The drawing under review shows one solid part. Ordinate dimensions are in mm from its lowest x, y, z. A direction names the side the tool comes from. Coordinates: 2 decimals unless noted, no trailing zeros. Write each loop counter-clockwise with the first axis right and the second up, starting at its lowest first coordinate (ties: lowest second). Pieces come first, ordered by that corner, then holes.
1) For line 1 (Y direction, x = 3.8, z = 5.4); line 2 (X direction, y = 5.25, z = 2.9); line 3 (Y direction, x = 1.3, z = 2.45), list the stretches that pass through material, from the lowest coordinate up.
2) Machinability: for the marked faces 1 and 2, which of the approach directions +Z, -Z, +X, -X, +Y, -Y give a long, thin tool a straight path to every point of the face, cutting with its end or side? Answer none if there is none.
3) Add section A-A, the plane y = 3.5. State the section outline as (x, z) points.
4) For P1, Ø1, axis at y = 7, z = 0.5, coming from the -X side; P2, Ø3, axis at x = 2, z = 4.5, coming from the -Y side; P3, Ø2, axis at x = 3, y = 7.5, coming from the +Z side, all flat-tipped, find the tip position at first contact; note any pin that passes through.
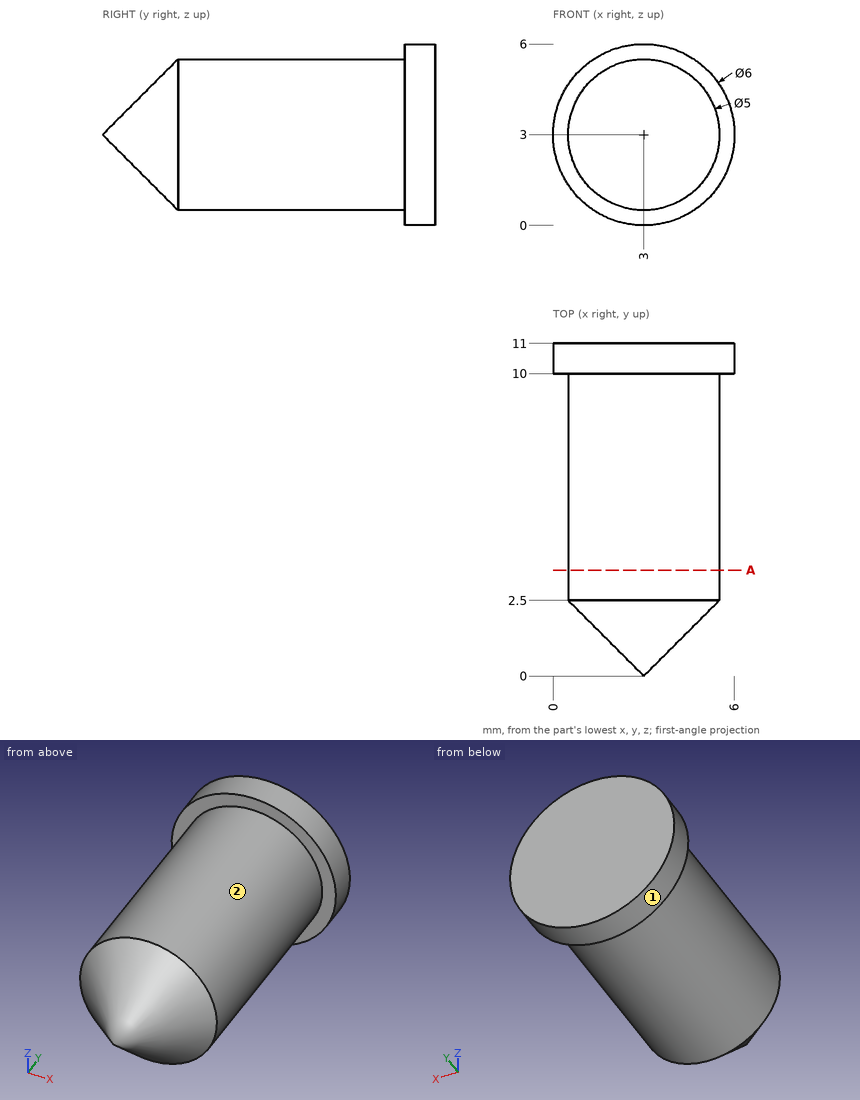
Geometry results:
1. line 1: y = 10 to 11
1. line 2: x = 0.5 to 5.5
1. line 3: y = 1.79 to 11
2. face 1: +Y, -Y
2. face 2: -Y
3. outline: circle Ø5 at (3, 3)
4. P1: stops at x = 1.5
4. P2: stops at y = 0.3
4. P3: stops at z = 5.5
